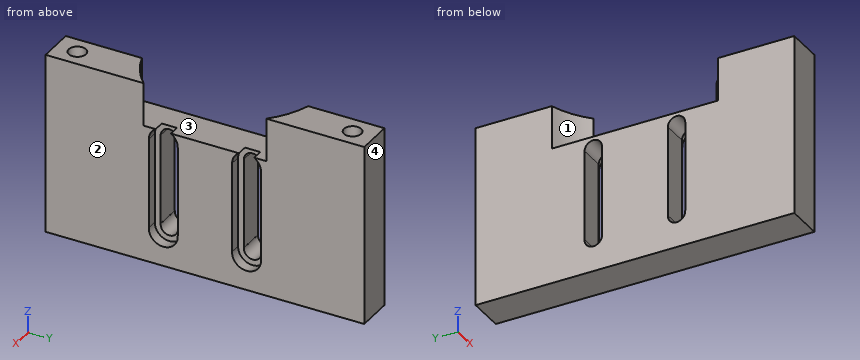
```python
from build123d import *

# Parameters (mm, degrees)
CYLINDER014_R             = 2
CYLINDER014_DEPTH         = 1.6
CYLINDER015_R             = 2
CYLINDER015_DEPTH         = 1.6
BOX003_W                  = 12.5
BOX003_H                  = 4
BOX003_DEPTH              = 1.6
FUSION006_PLACEMENT_ANGLE = 90
CYLINDER016_R             = 2
CYLINDER016_DEPTH         = 1.6
CYLINDER017_R             = 2
CYLINDER017_DEPTH         = 1.6
BOX004_W                  = 12.5
BOX004_H                  = 4
BOX004_DEPTH              = 1.6
FUSION007_PLACEMENT_ANGLE = 90
CYLINDER007_R             = 1.195
CYLINDER007_DEPTH         = 10
CYLINDER006_R             = 1.195
CYLINDER006_DEPTH         = 10
CYLINDER005_R             = 12
CYLINDER005_DEPTH         = 17
CYLINDER001_R             = 1.2
CYLINDER001_DEPTH         = 10
CYLINDER002_R             = 1.2
CYLINDER002_DEPTH         = 10
BOX001_W                  = 12.5
BOX001_H                  = 2.4
BOX001_DEPTH              = 10
FUSION_PLACEMENT_ANGLE    = 90
CYLINDER003_R             = 1.2
CYLINDER003_DEPTH         = 10
CYLINDER004_R             = 1.2
CYLINDER004_DEPTH         = 10
BOX002_W                  = 12.5
BOX002_H                  = 2.4
BOX002_DEPTH              = 10
FUSION001_PLACEMENT_ANGLE = 90
BOX_W                     = 5
BOX_H                     = 44
BOX_DEPTH                 = 25


with BuildPart() as cylinder014:
    # Cylinder014 → Cylinder014 (new body)
    with BuildSketch(Plane.XY):
        Circle(CYLINDER014_R)
    extrude(amount=CYLINDER014_DEPTH)


with BuildPart() as cylinder015:
    # Cylinder015 → Cylinder015 (new body)
    with BuildSketch(Plane(origin=(12.6, 0, 0), x_dir=(1, 0, 0), z_dir=(0, 0, 1))):
        Circle(CYLINDER015_R)
    extrude(amount=CYLINDER015_DEPTH)


with BuildPart() as langloch002:
    # Box003 → Box003 (new body)
    with BuildSketch(Plane(origin=(0, -2, 0), x_dir=(1, 0, 0), z_dir=(0, 0, 1))):
        with Locations((6.25, 2)):
            Rectangle(BOX003_W, BOX003_H)
    extrude(amount=BOX003_DEPTH)

    # Fusion006: union Cylinder014, Cylinder015
    add(cylinder014.part)
    add(cylinder015.part)


with BuildPart() as langloch002_1:
    # Fusion006 placement: moved
    add(langloch002.part.moved(Location((7, -5.75, -7.7))).rotate(Axis((7, -5.75, -7.7), (0, 1, 0)), FUSION006_PLACEMENT_ANGLE))


with BuildPart() as cylinder016:
    # Cylinder016 → Cylinder016 (new body)
    with BuildSketch(Plane.XY):
        Circle(CYLINDER016_R)
    extrude(amount=CYLINDER016_DEPTH)


with BuildPart() as cylinder017:
    # Cylinder017 → Cylinder017 (new body)
    with BuildSketch(Plane(origin=(12.6, 0, 0), x_dir=(1, 0, 0), z_dir=(0, 0, 1))):
        Circle(CYLINDER017_R)
    extrude(amount=CYLINDER017_DEPTH)


with BuildPart() as fusion008:
    # Box004 → Box004 (new body)
    with BuildSketch(Plane(origin=(0, -2, 0), x_dir=(1, 0, 0), z_dir=(0, 0, 1))):
        with Locations((6.25, 2)):
            Rectangle(BOX004_W, BOX004_H)
    extrude(amount=BOX004_DEPTH)

    # Fusion007: union Cylinder016, Cylinder017
    add(cylinder016.part)
    add(cylinder017.part)


with BuildPart() as fusion008_1:
    # Fusion007 placement: moved
    add(fusion008.part.moved(Location((7, 5.75, -7.7))).rotate(Axis((7, 5.75, -7.7), (0, 1, 0)), FUSION007_PLACEMENT_ANGLE))

    # Fusion008: union Langloch002
    add(langloch002_1.part)


with BuildPart() as cylinder007:
    # Cylinder007 → Cylinder007 (new body)
    with BuildSketch(Plane(origin=(6, -19, -8), x_dir=(1, 0, 0), z_dir=(0, 0, 1))):
        Circle(CYLINDER007_R)
    extrude(amount=CYLINDER007_DEPTH)


with BuildPart() as fusion003:
    # Cylinder006 → Cylinder006 (new body)
    with BuildSketch(Plane(origin=(6, 19, -8), x_dir=(1, 0, 0), z_dir=(0, 0, 1))):
        Circle(CYLINDER006_R)
    extrude(amount=CYLINDER006_DEPTH)

    # Fusion003: union Cylinder007
    add(cylinder007.part)


with BuildPart() as cylinder005:
    # Cylinder005 → Cylinder005 (new body)
    with BuildSketch(Plane.XY.offset(-6)):
        Circle(CYLINDER005_R)
    extrude(amount=CYLINDER005_DEPTH)


with BuildPart() as cylinder001:
    # Cylinder001 → Cylinder001 (new body)
    with BuildSketch(Plane.XY):
        Circle(CYLINDER001_R)
    extrude(amount=CYLINDER001_DEPTH)


with BuildPart() as cylinder002:
    # Cylinder002 → Cylinder002 (new body)
    with BuildSketch(Plane(origin=(12.6, 0, 0), x_dir=(1, 0, 0), z_dir=(0, 0, 1))):
        Circle(CYLINDER002_R)
    extrude(amount=CYLINDER002_DEPTH)


with BuildPart() as langloch:
    # Box001 → Box001 (new body)
    with BuildSketch(Plane(origin=(0, -1.2, 0), x_dir=(1, 0, 0), z_dir=(0, 0, 1))):
        with Locations((6.25, 1.2)):
            Rectangle(BOX001_W, BOX001_H)
    extrude(amount=BOX001_DEPTH)

    # Fusion: union Cylinder001, Cylinder002
    add(cylinder001.part)
    add(cylinder002.part)


with BuildPart() as langloch_1:
    # Fusion placement: moved
    add(langloch.part.moved(Location((0, 5.75, -7.7))).rotate(Axis((0, 5.75, -7.7), (0, 1, 0)), FUSION_PLACEMENT_ANGLE))


with BuildPart() as cylinder003:
    # Cylinder003 → Cylinder003 (new body)
    with BuildSketch(Plane.XY):
        Circle(CYLINDER003_R)
    extrude(amount=CYLINDER003_DEPTH)


with BuildPart() as cylinder004:
    # Cylinder004 → Cylinder004 (new body)
    with BuildSketch(Plane(origin=(12.6, 0, 0), x_dir=(1, 0, 0), z_dir=(0, 0, 1))):
        Circle(CYLINDER004_R)
    extrude(amount=CYLINDER004_DEPTH)


with BuildPart() as fusion002:
    # Box002 → Box002 (new body)
    with BuildSketch(Plane(origin=(0, -1.2, 0), x_dir=(1, 0, 0), z_dir=(0, 0, 1))):
        with Locations((6.25, 1.2)):
            Rectangle(BOX002_W, BOX002_H)
    extrude(amount=BOX002_DEPTH)

    # Fusion001: union Cylinder003, Cylinder004
    add(cylinder003.part)
    add(cylinder004.part)


with BuildPart() as fusion002_1:
    # Fusion001 placement: moved
    add(fusion002.part.moved(Location((0, -5.75, -7.7))).rotate(Axis((0, -5.75, -7.7), (0, 1, 0)), FUSION001_PLACEMENT_ANGLE))

    # Fusion002: union Langloch
    add(langloch_1.part)


with BuildPart() as obj1:
    # Box → Box (new body)
    with BuildSketch(Plane(origin=(3.5, -22, -25), x_dir=(1, 0, 0), z_dir=(0, 0, 1))):
        with Locations((2.5, 22)):
            Rectangle(BOX_W, BOX_H)
    extrude(amount=BOX_DEPTH)

    # Cut001: cut Fusion002
    add(fusion002_1.part, mode=Mode.SUBTRACT)

    # Cut002: cut Cylinder005
    add(cylinder005.part, mode=Mode.SUBTRACT)

    # Cut003: cut Fusion003
    add(fusion003.part, mode=Mode.SUBTRACT)

    # Cut006: cut Fusion008
    add(fusion008_1.part, mode=Mode.SUBTRACT)


solid = obj1.part
```
Work out the finished part from the listing and answer in its coordinate system (mm). Face numbers are marked on the shaded views. Give positions to 0.01 mm unless a question says otherwise; leave off trailing zeros. Order: outer loops, then holes, each group sorted by start corner. A loop starts at its lowest first (then second) coordinate and runs counter-clockwise, first axis right, second up. Notation, with made-up numbers: (-14.5, 3) - (44.5, 3) arc R14 ccw to (44.5, 9) - close; hole circle Ø6 at (59.5, -11). An arc over 180 degrees is marked (long way). One line per item, written item: value. Start each with the question number.
1. Section D-D, the plane x = 6.5 is taken. Count the separate pieces of the cut face and the enclosed holes in it, then the cut area to 3 significant figures.
2. Consider line 1 (Y direction, x = 5.6, z = -14.5); line 2 (X direction, y = -19, z = -1.5) (3 decimals). Determine where each line is inside the solid, lowest interval first.
3. Section C-C, the plane z = -9.5 is taken. Write down the section's boundary in (x, y).
4. Section A-A, the plane y = 5.75 is taken. Write down the section's boundary in (x, z), then the cut area to 4 significant figures.
5. Section B-B, the plane z = -3.5 is taken. Write down the section's boundary in (x, y) (3 decimals), then the cut area to 3 significant figures.
6. Each of these flat-tipped pins is pushed along its axis until it touches: pin 1 Ø1.2 at (x, y) = (6, 18.5) entering from +Z; pin 2 Ø2 at (y, z) = (-6, -13.5) entering from +X; pin 3 Ø1.9 at (y, z) = (5.75, -20.3) entering from +X. Where does it stop, or does it pass through?
7. For a pull along Y with two mould halves and no side action, classify the marked faces 1, 2, 3 and 4 as released by +Y, released by -Y, zero draft, split by the parting line, or undercut.
Filled sheet:
1. separate pieces: 1
1. enclosed holes: 2
1. area: 875 mm²
2. line 1: -22 to -6.95, -4.55 to 4.55, 6.95 to 22
2. line 2: 3.5 to 4.805, 7.195 to 8.5
3. outline: (3.5, -22) - (8.5, -22) - (8.5, -7.75) - (7, -7.75) - (7, -6.95) - (3.5, -6.95) - close; (3.5, -4.55) - (7, -4.55) - (7, -3.75) - (8.5, -3.75) - (8.5, 3.75) - (7, 3.75) - (7, 4.55) - (3.5, 4.55) - close; (3.5, 6.95) - (7, 6.95) - (7, 7.75) - (8.5, 7.75) - (8.5, 22) - (3.5, 22) - close
4. outline: (3.5, -25) - (8.5, -25) - (8.5, -22.3) - (7, -22.3) - (7, -21.5) - (3.5, -21.5) - close; (3.5, -6.5) - (7, -6.5) - (7, -6) - (3.5, -6) - close
4. area: 18.05 mm²
5. outline: (3.5, -22) - (8.5, -22) - (8.5, -8.471) arc R12 cw to (3.5, -11.478) - close; (3.5, 11.478) arc R12 cw to (8.5, 8.471) - (8.5, 22) - (3.5, 22) - close; hole circle Ø2.39 at (6, -19); hole circle Ø2.39 at (6, 19)
5. area: 108 mm²
6. pin 1: z = -8
6. pin 2: x = 7
6. pin 3: through
7. face 1: undercut
7. face 2: zero draft
7. face 3: undercut
7. face 4: released by +Y
